Part model, mm, in its own coordinate system. Face numbers are marked on the shaded views. Round coordinates to 2 decimals unless told otherwise and drop trailing zeros. Write each loop counter-clockwise with the first axis right and the second up, starting at its lowest first coordinate (ties: lowest second). Pieces come first, ordered by that corner, then holes. Notation, with made-up numbers: (19, -36) -> (62, -36) arc R17 cw to (62, -15) -> close; hole circle Ø8 at (-22, 27.25). An arc over 180 degrees is marked (long way). Use CSV: the item, a comma, the result in double quotes. Start each with the question number.
(1) Probe line 1 (X direction, y = 3.75, z = 75.25); line 2 (X direction, y = 1.5, z = 0); line 3 (X direction, y = 1.25, z = 73). List the from-to ranges inside material, lowest first. Write a range as [from, to].
(2) Saw through at B-B (z = 0). Give the cut face in (x, y).
(3) Drop a flat-ended pin along its axis: pin 1 (10 mm diameter, centred on x = 24.5, z = -60, fed in from -Y). Give the stop position or say it passes through.
(4) Saw through at A-A (x = 0). Give the cut face in (y, z), plus the area to 3 significant figures.
(5) Saw through at C-C (y = 2.5). Give the cut face in (x, z), plus the area to 3 significant figures.
(6) Two-plate mould, pull along Y, no slides. Class the marked faces 1 and 2: released by +Y, released by -Y, zero draft, split by the parting line, or undercut.
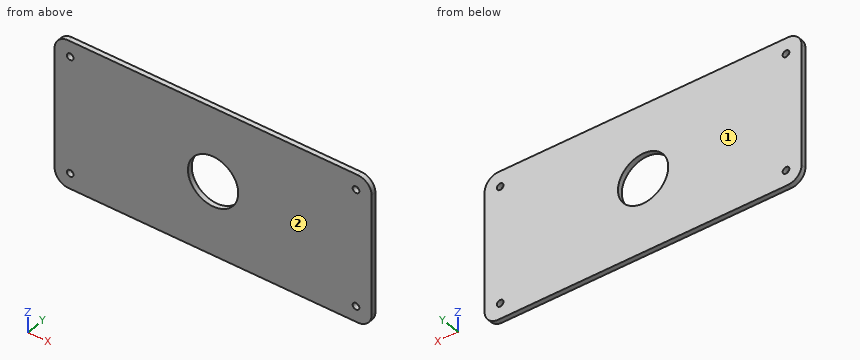
```python
from build123d import *

# Parameters (mm, degrees)
SKETCH1_W           = 406.4
SKETCH1_H           = 190.5
BOSS_EXTRUDE1_DEPTH = 6.35
SKETCH2_R           = 32.25
CUT_EXTRUDE1_DEPTH  = 225.506403027
SKETCH3_R           = 4.25
CUT_EXTRUDE2_DEPTH  = 225.506403027
FILLET1_R           = 17.78


with BuildPart() as part:
    # Sketch1 → Boss-Extrude1 (new body)
    with BuildSketch(Plane(origin=(0, 0, 0), x_dir=(1, 0, 0), z_dir=(0, 1, 0))):
        Rectangle(SKETCH1_W, SKETCH1_H)
    extrude(amount=BOSS_EXTRUDE1_DEPTH)

    # Sketch2 → Cut-Extrude1 (cut, through all)
    with BuildSketch(Plane(origin=(0, 6.35, 0), x_dir=(1, 0, 0), z_dir=(0, 1, 0))):
        with Locations(Location((0, 0, 0), (0, 0, 270))):
            Circle(SKETCH2_R)
    extrude(amount=-CUT_EXTRUDE1_DEPTH, mode=Mode.SUBTRACT)

    # Sketch3 → Cut-Extrude2 (cut, through all)
    with BuildSketch(Plane(origin=(0, 6.35, 0), x_dir=(1, 0, 0), z_dir=(0, 1, 0))):
        with Locations(Location((-183.2, 75.25, 0), (0, 0, 270))):
            Circle(SKETCH3_R)
        with Locations(Location((183.2, 75.25, 0), (0, 0, 270))):
            Circle(SKETCH3_R)
        with Locations(Location((183.2, -75.25, 0), (0, 0, 270))):
            Circle(SKETCH3_R)
        with Locations(Location((-183.2, -75.25, 0), (0, 0, 270))):
            Circle(SKETCH3_R)
    extrude(amount=-CUT_EXTRUDE2_DEPTH, mode=Mode.SUBTRACT)

    # Fillet1
    fillet1_edges = [part.edges().sort_by_distance(p)[0] for p in [
        (203.2, 3.175, 95.25),
        (-203.2, 3.175, 95.25),
        (-203.2, 3.175, -95.25),
        (203.2, 3.175, -95.25),
    ]]
    fillet(fillet1_edges, radius=FILLET1_R)


solid = part.part
```
Answers:
1,line 1,"x = [-203.2, -187.45], [-178.95, 178.95], [187.45, 203.2]"
1,line 2,"x = [-203.2, -32.25], [32.25, 203.2]"
1,line 3,"x = [-203.2, -186.81], [-179.59, 179.59], [186.81, 203.2]"
2,outline,"(-203.2, 0) -> (-32.25, 0) -> (-32.25, 6.35) -> (-203.2, 6.35) -> close; (32.25, 0) -> (203.2, 0) -> (203.2, 6.35) -> (32.25, 6.35) -> close"
3,pin 1,"stops at y = 0"
4,outline,"(0, -95.25) -> (6.35, -95.25) -> (6.35, -32.25) -> (0, -32.25) -> close; (0, 32.25) -> (6.35, 32.25) -> (6.35, 95.25) -> (0, 95.25) -> close"
4,area,"800 mm²"
5,outline,"(-203.2, -77.47) arc R17.78 ccw to (-185.42, -95.25) -> (185.42, -95.25) arc R17.78 ccw to (203.2, -77.47) -> (203.2, 77.47) arc R17.78 ccw to (185.42, 95.25) -> (-185.42, 95.25) arc R17.78 ccw to (-203.2, 77.47) -> close; hole circle Ø8.5 at (-183.2, -75.25); hole circle Ø8.5 at (-183.2, 75.25); hole circle Ø64.5 at (0, 0); hole circle Ø8.5 at (183.2, -75.25); hole circle Ø8.5 at (183.2, 75.25)"
5,area,"73,700 mm²"
6,face 1,"released by +Y"
6,face 2,"released by -Y"
